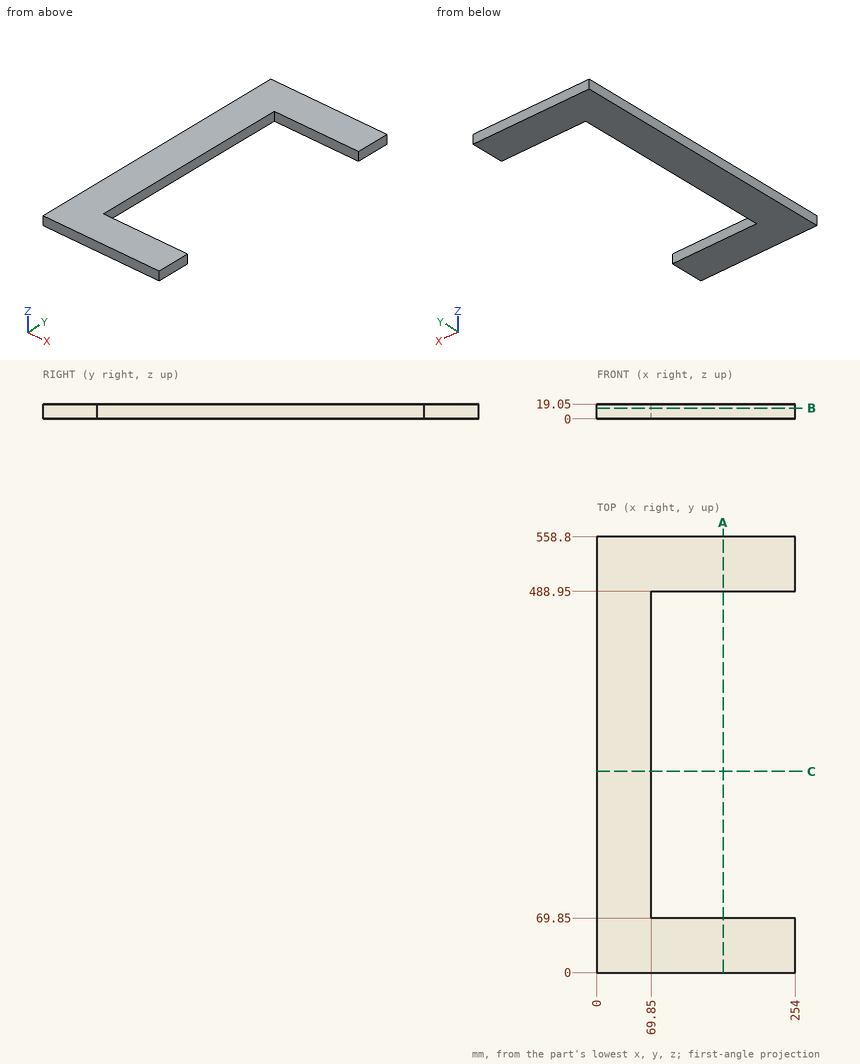
For this review, use the dimensioned drawing (mm, ordinates from the lowest corner) and the shaded views. Round coordinates to 2 decimals unless told otherwise and drop trailing zeros. Write each loop counter-clockwise with the first axis right and the second up, starting at its lowest first coordinate (ties: lowest second). Pieces come first, ordered by that corner, then holes. Notation, with made-up numbers: (65, 9.5) -> (122, 9.5) arc R19 ccw to (122, 20.5) -> close; hole circle Ø9 at (28, -34). An arc over 180 degrees is marked (long way). Use CSV: the item, a comma, the result in double quotes.
Q1. Consider section A-A (x = 162). Give the boundary of the cut face in (y, z), then the cut area to 3 significant figures.
Checks:
outline,"(0, 0) -> (69.85, 0) -> (69.85, 19.05) -> (0, 19.05) -> close; (488.95, 0) -> (558.8, 0) -> (558.8, 19.05) -> (488.95, 19.05) -> close"
area,"2,660 mm²"
Q2. For pin 1 Ø9.5 at (y, z) = (178, 10.5) entering from +X, flat-tipped, find the tip position at first contact; note if it passes through.
Checks:
pin 1,"x = 69.85"
Q3. Consider section B-B (z = 13.75). Give the boundary of the cut face in (x, y).
Checks:
outline,"(0, 0) -> (254, 0) -> (254, 69.85) -> (69.85, 69.85) -> (69.85, 488.95) -> (254, 488.95) -> (254, 558.8) -> (0, 558.8) -> close"
Q4. To check wall thickness, follow probe 1 along Y at (x, z) = (115, 12.5); probe 2 along X at (y, z) = (339, 16.5). State the ranges of each line that lie inside material, in increasing order. Write a range as [from, to].
Checks:
probe 1,"[0, 69.85], [488.95, 558.8]"
probe 2,"[0, 69.85]"
Q5. Consider section C-C (y = 258). Give the boundary of the cut face in (x, z).
Checks:
outline,"(0, 0) -> (69.85, 0) -> (69.85, 19.05) -> (0, 19.05) -> close"
